Check sheet for the modelled part. Datum: model origin and axes. Units: mm. Face numbers are marked on the shaded views. Give positions to 0.01 mm unless a question says otherwise; leave off trailing zeros. Order: outer loops, then holes, each group sorted by start corner. A loop starts at its lowest first (then second) coordinate and runs counter-clockwise, first axis right, second up.
Item 1: Sectioned sample at A-A on x = 6. Record the boundary of the cut face in (y, z).
Item 2: Release check for a two-part mould opening along Y. For the marked faces 1 and 2 record: released by +Y, released by -Y, zero draft, split by the parting line, or undercut.
Item 3: Sectioned sample at B-B on z = -4.75. Count the separate pieces of the cut face and the enclosed holes in it, and give its area (3 significant figures).
Item 4: Sectioned sample at D-D on x = -85. Record the boundary of the cut face in (y, z), and give its area (4 significant figures).
Item 5: Material ranges on line 1 along Y through (x, z) = (0, -5.85); line 2 along X through (y, z) = (-6, -0.25); line 3 along X through (y, z) = (-36, -0.75), recorded low to high.
Item 6: Gauge pin test, flat ends, axial feed: P1, Ø10, axis at x = -22.5, y = -63, coming from the +Z side; P2, Ø2, axis at y = -81.5, z = -5.5, coming from the -X side; P3, Ø20.5, axis at x = 7.5, y = -6, coming from the -Z side; P4, Ø5, axis at x = -9, z = -5, coming from the +Y side. Record the tip position at first contact, or that the pin passes through.
Item 7: Sectioned sample at C-C on y = -78.5. Record the boundary of the cut face in (x, z).
from build123d import *

# Parameters (mm, degrees)
SKETCH1_R           = 2.5
BOSS_EXTRUDE1_DEPTH = 12
CUT_EXTRUDE2_DEPTH  = 5
SKETCH2_R           = 20.406966807
SKETCH2_R_2         = 18.406966807
CUT_EXTRUDE1_DEPTH  = 5


with BuildPart() as part:
    # Sketch1 → Boss-Extrude1 (new body)
    with BuildSketch(Plane.XY):
        with BuildLine():
            Line((-26.955627075, 25.359398414), (44.050751749, 70.198338512))
            add(Edge.make_bspline(
                [(44.050751749, 70.198338512), (62.087157858, 60.129124735), (102.236821697, -14.309839041), (30.255220871, -56.610877482)],
                knots=[0, 0, 0, 0, 1, 1, 1, 1], degree=3))
            Line((30.255220871, -56.610877482), (-92.542495842, -130.724182913))
            Line((-92.542495842, -130.724182913), (-109.546280871, -97.192243206))
            Line((-109.546280871, -97.192243206), (-53.551819625, -58.475967995))
            ThreePointArc((-53.551819625, -58.475967995), (-44.950344781, -47.729789478), (-43.667906214, -34.025006607))
            Line((-43.667906214, -34.025006607), (-55.484471769, 25.012678553))
            ThreePointArc((-55.484471769, 25.012678553), (-55.229156607, 26.186005417), (-54.194896814, 26.796077907))
            Line((-54.194896814, 26.796077907), (-36.765460017, 28.917713338))
            Line((-36.765460017, 28.917713338), (-34.712668517, 26.525380142))
            ThreePointArc((-34.712668517, 26.525380142), (-31.051074716, 24.4992182), (-26.955627075, 25.359398414))
        make_face()
        Circle(SKETCH1_R, mode=Mode.SUBTRACT)
        with BuildLine():
            Line((38.077539086, 8.627342387), (31.457970773, 37.843392922))
            ThreePointArc((31.457970773, 37.843392922), (36.113405951, 45.226418252), (43.49643128, 40.570983074))
            Line((43.49643128, 40.570983074), (50.115999593, 11.354932539))
            ThreePointArc((50.115999593, 11.354932539), (47.829544092, -18.785170217), (28.993629861, -42.425432651))
            Line((28.993629861, -42.425432651), (-1.139071825, -63.018184329))
            ThreePointArc((-1.139071825, -63.018184329), (-9.716926906, -61.404944758), (-8.103687335, -52.827089677))
            Line((-8.103687335, -52.827089677), (22.029014352, -32.234337999))
            ThreePointArc((22.029014352, -32.234337999), (36.340317452, -14.272748403), (38.077539086, 8.627342387))
        make_face(mode=Mode.SUBTRACT)
    extrude(amount=-BOSS_EXTRUDE1_DEPTH)

    # Sketch3 → Cut-Extrude2 (cut)
    with BuildSketch(Plane(origin=(0, 0, -12), x_dir=(-1, 0, 0), z_dir=(0, 0, -1))):
        with BuildLine():
            Line((108.633361408, -98.992545924), (93.449492386, -128.935560359))
            Line((93.449492386, -128.935560359), (91.732523821, -127.89930155))
            Line((91.732523821, -127.89930155), (-29.231808811, -54.892516323))
            add(Edge.make_bspline(
                [(-44.065734477, 67.842412696), (-44.711989199, 67.409412256), (-45.319058391, 66.940521732), (-46.487121265, 65.960540056), (-47.04734625, 65.448744854), (-48.676831708, 63.866474713), (-49.695652132, 62.74980166), (-51.643061578, 60.433812481), (-52.570637695, 59.233568633), (-54.351661803, 56.76518688), (-55.206220539, 55.494184071), (-57.642169465, 51.637395526), (-59.108475151, 48.994377471), (-61.772216068, 43.585851359), (-62.968525898, 40.819830599), (-64.562191776, 36.579321004), (-65.059713989, 35.150465126), (-65.753925807, 32.983458962), (-65.976639631, 32.257164595), (-66.404295719, 30.796479627), (-66.609516748, 30.060994816), (-67.585549406, 26.379930292), (-68.207997329, 23.421535241), (-69.124162601, 17.476634327), (-69.417856055, 14.49012642), (-69.647875237, 8.486550939), (-69.584312973, 5.469492942), (-69.186185446, 0.918013899), (-69.001954276, -0.606436507), (-68.53395704, -3.614530288), (-68.249900615, -5.10403396), (-67.246805131, -9.528696616), (-66.377032654, -12.420063251), (-64.763908669, -16.667495261), (-64.174739481, -18.06835499), (-63.212508348, -20.146844678), (-62.87805617, -20.837039742), (-62.187699389, -22.200245629), (-61.831475952, -22.874060854), (-59.996492333, -26.20515645), (-58.3564207, -28.748698204), (-54.76187252, -33.614098874), (-52.807325031, -35.935907769), (-49.657387027, -39.264829798), (-48.576129174, -40.343226595), (-46.36681057, -42.431345516), (-45.23699415, -43.442927339), (-39.471767159, -48.350894333), (-34.491238963, -51.801735421), (-29.231808811, -54.892516323)],
                knots=[0, 0, 0, 0, 0.015625, 0.015625, 0.03125, 0.03125, 0.0625, 0.0625, 0.09375, 0.09375, 0.125, 0.125, 0.1875, 0.1875, 0.25, 0.25, 0.28125, 0.28125, 0.296875, 0.296875, 0.3125, 0.3125, 0.375, 0.375, 0.4375, 0.4375, 0.5, 0.5, 0.53125, 0.53125, 0.5625, 0.5625, 0.625, 0.625, 0.65625, 0.65625, 0.671875, 0.671875, 0.6875, 0.6875, 0.75, 0.75, 0.8125, 0.8125, 0.84375, 0.84375, 0.875, 0.875, 1, 1, 1, 1], degree=3))
            Line((-44.065734477, 67.842412696), (25.887763568, 23.668343261))
            ThreePointArc((25.887763568, 23.668343261), (31.348360423, 22.521436309), (36.230485491, 25.222985565))
            Line((36.230485491, 25.222985565), (37.586279366, 26.80303434))
            Line((37.586279366, 26.80303434), (53.417437888, 24.875952746))
            Line((53.417437888, 24.875952746), (41.706802558, -33.632485968))
            ThreePointArc((41.706802558, -33.632485968), (43.096111006, -48.479334078), (52.414375421, -60.121027471))
            Line((52.414375421, -60.121027471), (106.973050581, -97.844556472))
            Line((106.973050581, -97.844556472), (108.633361408, -98.992545924))
        make_face()
    extrude(amount=-CUT_EXTRUDE2_DEPTH, mode=Mode.SUBTRACT)

    # Sketch2 → Cut-Extrude1 (cut)
    with BuildSketch(Plane(origin=(0, 0, -7), x_dir=(-1, 0, 0), z_dir=(0, 0, -1))):
        Circle(SKETCH2_R)
        Circle(SKETCH2_R_2, mode=Mode.SUBTRACT)
    extrude(amount=-CUT_EXTRUDE1_DEPTH, mode=Mode.SUBTRACT)


solid = part.part
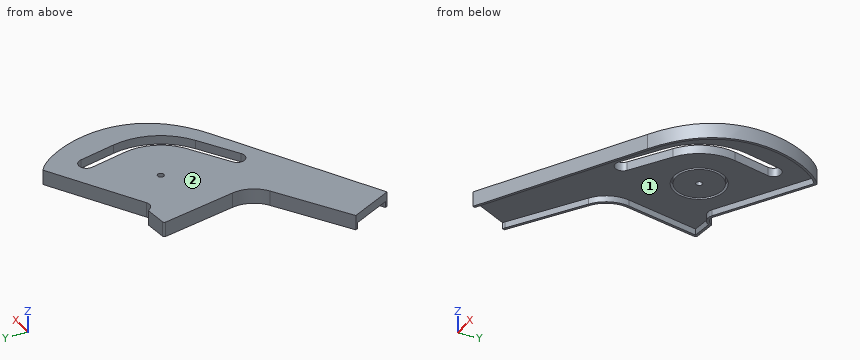
Report:
1. outline: (-71.25, -12) - (-68.91, -12) - (-68.91, -7) - (-58.14, -7) - (-58.14, 0) - (-71.25, 0) - close; (-43.19, -7) - (-19.5, -7) - (-19.5, -2) - (-17.4, -2) - (-17.4, -7) - (17.4, -7) - (17.4, -2) - (19.5, -2) - (19.5, -7) - (43.8, -7) - (43.8, -12) - (46.17, -12) - (46.17, 0) - (-43.19, 0) - close
2. face 1: undercut
2. face 2: zero draft
3. separate pieces: 2
3. enclosed holes: 3
3. area: 13,900 mm2
4. outline: (-126.17, -12) - (-123.84, -12) - (-123.84, -7) - (-82.65, -7) - (-82.65, -12) - (-80.22, -12) - (-80.22, 0) - (-126.17, 0) - close
4. area: 345.5 mm2
5. line 1: y = -74.87 to -62.24, -47.29 to -20.41, -18.41 to -2.5, 2.5 to 18.41, 20.41 to 42.38
5. line 2: x = -49.28 to 38.58, 51.03 to 70.09
5. line 3: x = -43.36 to 16.52, 36.67 to 55.31
6. P1: stops at z = 0
6. P2: stops at x = -88.3
6. P3: stops at z = -7
6. P4: stops at y = 38.28
7. outline: (-82.51, -12) - (-79, -12) - (-79, -7) - (-9.88, -7) - (-9.88, -12) - (-6.01, -12) - (-6.01, 0) - (-82.51, 0) - close
